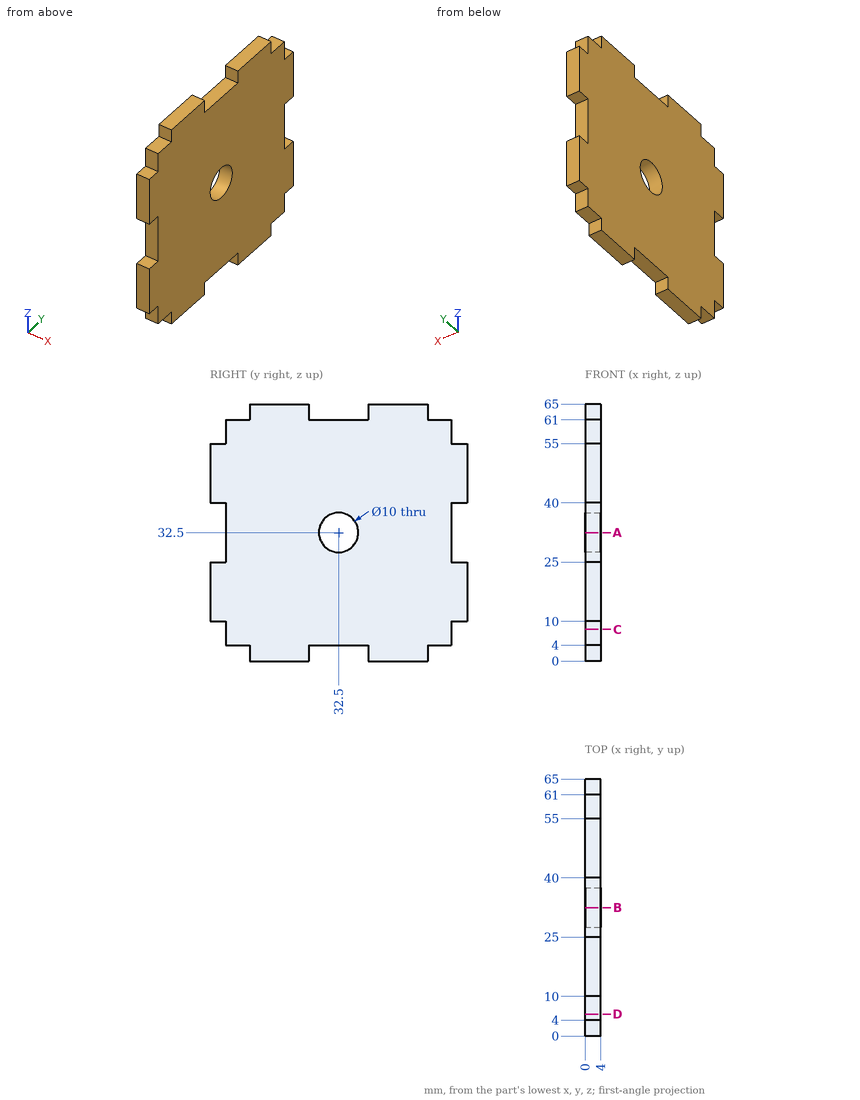
Study the drawing (mm; zero at the part's minimum x, y, z) and answer. Round coordinates to 2 decimals unless told otherwise and drop trailing zeros. Order: outer loops, then holes, each group sorted by start corner. A loop starts at its lowest first (then second) coordinate and runs counter-clockwise, first axis right, second up. Notation, with made-up numbers: M 82.5,-9.5 L 93.5,-9.5 A17 ccw 93.5,14.5 Z; hole C -4,19.25 d8. An arc over 180 degrees is marked long. One line per item, written item: value.
Q1. Straight lines are drawn through the part: line 1 (Y direction, x = 2.4, z = 32.5); line 2 (Z direction, x = 1.05, y = 26.5). For each, find the intervals that lie inside material, in ascending order.
Derived:
line 1: 4 to 27.5, 37.5 to 61
line 2: 4 to 61
Q2. Flat-ended cylindrical pins translate along their axes: pin 1 (4 mm diameter, centred on y = 28, z = 11.5, fed in from -X); pin 2 (1.2 mm diameter, centred on x = 2, y = 1, fed in from -Z); pin 3 (1.2 mm diameter, centred on x = 2, z = 7, fed in from -Y); pin 4 (2 mm diameter, centred on x = 1.5, z = 7.5, fed in from +Y). Find the tip coordinate at first contact, or state that the pin passes through.
Derived:
pin 1: x = 0
pin 2: z = 10
pin 3: y = 4
pin 4: y = 61
Q3. Find section A-A on z = 32.5. Write down the section's boundary in (x, y).
Derived:
outline: M 0,4 L 4,4 L 4,27.5 L 0,27.5 Z; M 0,37.5 L 4,37.5 L 4,61 L 0,61 Z
Q4. Find section C-C on z = 8. Write down the section's boundary in (x, y).
Derived:
outline: M 0,4 L 4,4 L 4,61 L 0,61 Z
